Work out the finished part from the listing and answer in its coordinate system (mm). A direction names the side the tool comes from. Round coordinates to 2 decimals unless told otherwise and drop trailing zeros. Loops run counter-clockwise (first coordinate to the right, second up) from the corner with the lowest first, then second, coordinate; pieces in that order, holes last. Notation, with made-up numbers: (29, -0.75) - (50, -0.75) arc R6 cw to (50, 8.25) - close; hole circle Ø10 at (51.5, -23). An arc over 180 degrees is marked (long way). Answer as CSV lines item,"result". Start each with the question number.
```python
from build123d import *

# Parameters (mm, degrees)
F0_W      = 107.95
F0_H      = 63.5
F1_DEPTH  = 57.15
F2_W      = 6.35
F2_H      = 6.35
F3_DEPTH  = 57.151
F4_W      = 63.5
F4_H      = 12.7
F5_DEPTH  = 57.151
F6_W      = 31.7601591736
F6_H      = 31.75
F7_DEPTH  = 107.951
F8_W      = 12.7
F8_H      = 12.7
F9_DEPTH  = 31.75
F10_W     = 50.8
F10_H     = 12.7
F11_DEPTH = 31.75
F13_DEPTH = 57.151
F15_DEPTH = 50.801
F16_R     = 6.35
F17_DEPTH = 25.3908408264
F18_W     = 50.8
F18_H     = 31.75
F19_DEPTH = 19.051


with BuildPart() as f1:
    # F0 (on Front) → F1 (new body)
    with BuildSketch(Plane.XZ):
        with Locations((53.975, 31.75)):
            Rectangle(F0_W, F0_H)
    extrude(amount=F1_DEPTH)

    # F2 (on face) → F3 (cut, through all)
    with BuildSketch(Plane.XZ.offset(57.15)):
        with Locations((3.175, 3.175)):
            Rectangle(F2_W, F2_H)
    extrude(amount=-F3_DEPTH, mode=Mode.SUBTRACT)

    # F4 (on face) → F5 (cut, through all)
    with BuildSketch(Plane.XZ.offset(57.15)):
        with Locations((76.2, 6.35)):
            Rectangle(F4_W, F4_H)
    extrude(amount=-F5_DEPTH, mode=Mode.SUBTRACT)

    # F6 (on face) → F7 (cut, through all)
    with BuildSketch(Plane.YZ.offset(107.95)):
        with Locations((-41.2699204132, 47.625)):
            Rectangle(F6_W, F6_H)
    extrude(amount=-F7_DEPTH, mode=Mode.SUBTRACT)

    # F8 (on face) → F9 (cut)
    with BuildSketch(Plane.XZ.offset(57.15)):
        with Locations((50.8, 25.4)):
            Rectangle(F8_W, F8_H)
    extrude(amount=-F9_DEPTH, mode=Mode.SUBTRACT)

    # F10 (on face) → F11 (cut)
    with BuildSketch(Plane.XZ.offset(57.15)):
        with Locations((82.55, 25.4)):
            Rectangle(F10_W, F10_H)
    extrude(amount=-F11_DEPTH, mode=Mode.SUBTRACT)

    # F12 (on face) → F13 (cut, through all)
    with BuildSketch(Plane(origin=(0, 0, 0), x_dir=(-1, 0, 0), z_dir=(0, 1, 0))):
        Polygon((-107.95, 63.5), (-107.95, 31.75), (-50.8, 63.5), align=None)
    extrude(amount=-F13_DEPTH, mode=Mode.SUBTRACT)

    # F14 (on face) → F15 (cut, through all)
    with BuildSketch(Plane(origin=(0, 0, 12.7), x_dir=(1, 0, 0), z_dir=(0, 0, -1))):
        Polygon((92.075, 0), (107.95, 0), (107.95, 15.875), align=None)
    extrude(amount=-F15_DEPTH, mode=Mode.SUBTRACT)

    # F16 (on face) → F17 (cut, through all)
    with BuildSketch(Plane.XZ.offset(25.3898408264)):
        with Locations((19.05, 50.8)):
            Circle(F16_R)
    extrude(amount=-F17_DEPTH, mode=Mode.SUBTRACT)

    # F18 (on face) → F19 (cut, through all)
    with BuildSketch(Plane.XY.offset(19.05)):
        with Locations((82.55, -41.275)):
            Rectangle(F18_W, F18_H)
    extrude(amount=-F19_DEPTH, mode=Mode.SUBTRACT)


solid = f1.part
```
Item 1: Section A-A, the plane z = 50.8 is taken. Give the vertices of the cut face in (x, y).
Item 2: Determine the mould class of faces 4 (the face through (22.464, -12.873, 56.154)), 5 (the face through (107.95, -21, 22)), 6 (the face through (69, -23, 12.7)), 7 (the face through (25, -13, 63.5)) for opening direction Z: pulls with the +Z half, pulls with the -Z half, needs draft (parallel to the pull), parting line crosses it, or undercut.
Item 3: Find the intervals of material crossed by L1, parallel to X at y = -38.5, z = 16.5; L2, parallel to Z at x = 19.05, y = -8.25; L3, parallel to Y at x = 27.5, z = 42, in increasing order.
Item 4: Section B-B, the plane x = 19.05 is taken. Give the vertices of the cut face in (y, z), and give its area (3 significant figures).
Item 5: Flat-ended cylindrical pins translate along their axes: pin 1 Ø8 at (x, z) = (32, 39.5) entering from -Y; pin 2 Ø10 at (x, z) = (19.05, 50.8) entering from -Y; pin 3 Ø4 at (x, y) = (49, -42) entering from +Z; pin 4 Ø3 at (y, z) = (-23, 4) entering from -X. Find the tip coordinate at first contact, or state that the pin passes through.
Item 6: Which of the six approach directions +Z, -Z, +X, -X, +Y, -Y give full straight-line access (tool end or side, diameter ignored) to faces 1 (the face through (44.45, -41, 25)), 2 (the face through (3, -29, 6.35)), 3 (the face through (31, -41, 31.75))?
Item 7: Section C-C, the plane y = -45.5 is taken. Give the vertices of the cut face in (x, z).
Item 8: Section D-D, the plane z = 27 is taken. Give the vertices of the cut face in (x, y) (3 decimals), and give its area (3 significant figures).
Answer:
1,outline,"(0, -25.39) - (12.7, -25.39) - (12.7, 0) - (0, 0) - close; (25.4, -25.39) - (73.66, -25.39) - (73.66, 0) - (25.4, 0) - close"
2,face 4,"undercut"
2,face 5,"needs draft"
2,face 6,"pulls with the -Z half"
2,face 7,"pulls with the +Z half"
3,L1,"x = 0 to 57.15"
3,L2,"z = 0 to 44.45, 57.15 to 63.5"
3,L3,"y = -25.39 to 0"
4,outline,"(-57.15, 0) - (0, 0) - (0, 44.45) - (-25.39, 44.45) - (-25.39, 31.75) - (-57.15, 31.75) - close; (-25.39, 57.15) - (0, 57.15) - (0, 63.5) - (-25.39, 63.5) - close"
4,area,"2,300 mm²"
5,pin 1,"stops at y = -25.39"
5,pin 2,"passes through"
5,pin 3,"stops at z = 19.05"
5,pin 4,"stops at x = 6.35"
6,face 1,"+Z, +X, -Y"
6,face 2,"-Z, -X, +Y, -Y"
6,face 3,"+Z, +X, -X, -Y"
7,outline,"(0, 6.35) - (6.35, 6.35) - (6.35, 0) - (44.45, 0) - (44.45, 12.7) - (57.15, 12.7) - (57.15, 19.05) - (44.45, 19.05) - (44.45, 31.75) - (0, 31.75) - close"
8,outline,"(0, -57.15) - (44.45, -57.15) - (44.45, -25.4) - (107.95, -25.4) - (107.95, -15.875) - (92.075, 0) - (0, 0) - close"
8,area,"4,030 mm²"
